from build123d import *

# Parameters (mm, degrees)
SKETCH1_R           = 63.5
SKETCH1_R_2         = 38.1
BOSS_EXTRUDE1_DEPTH = 9.525
SKETCH2_R           = 66.04
SKETCH2_R_2         = 63.5
BOSS_EXTRUDE2_DEPTH = 1.27


with BuildPart() as part:
    # Sketch1 → Boss-Extrude1 (new, symmetric)
    with BuildSketch(Plane.XY):
        with Locations(Location((0, 0, 0), (0, 0, 180))):
            Circle(SKETCH1_R)
        with Locations(Location((0, 0, 0), (0, 0, 180))):
            Circle(SKETCH1_R_2, mode=Mode.SUBTRACT)
    extrude(amount=BOSS_EXTRUDE1_DEPTH, both=True)

    # Sketch2 → Boss-Extrude2 (add, symmetric)
    with BuildSketch(Plane.XY.offset(9.525)):
        Circle(SKETCH2_R)
        with Locations(Location((0, 0, 0), (0, 0, 180))):
            Circle(SKETCH2_R_2, mode=Mode.SUBTRACT)
    extrude(amount=BOSS_EXTRUDE2_DEPTH, both=True)


solid = part.part
Can you work these out from the model? Positions are in its coordinate system, mm. A direction names the side the tool comes from. Give positions to 0.01 mm unless a question says otherwise; leave off trailing zeros. Order: outer loops, then holes, each group sorted by start corner. A loop starts at its lowest first (then second) coordinate and runs counter-clockwise, first axis right, second up. Notation, with made-up numbers: M 42,64.25 L 76,64.25 A17 cw 76,97.25 Z; hole C 34,-17 d3. An arc over 180 degrees is marked long. Use a Markdown table: item, result. Add a question column.
Item 1: For faces 1 (the cylindrical face through (13.77, 61.99, -0.51)), 2 (the flat face through (-27.3, 27.3, -9.525)), 3 (the flat face through (-27.3, 27.3, 9.525)), which set-ups out of +Z, -Z, +X, -X, +Y, -Y let a thin tool reach every point of the face, with its end or its side?
Item 2: If I drill on L1, parallel to Y at x = 0, z = -1.5; L2, parallel to Y at x = 0, z = 9.85; L3, parallel to X at y = 1, z = -1.75, over which ranges is the centre line in solid material (lowest first)? Write a range as [from, to].
Item 3: Will these pins go through, and if not, where does the flat tip stop? pin 1 (5 mm diameter, centred on x = 28, z = -6, fed in from +Y); pin 2 (4 mm diameter, centred on x = -24.5, y = 27.5, fed in from +Z) (3 decimals); pin 3 (4 mm diameter, centred on y = 15, z = -0.5, fed in from +X).
Item 4: Suppose I cut it at A-A (y = 0). List the corners of the cut face in (x, z) for me (3 decimals).
Item 5: Suppose I cut it at C-C (z = 4.5). List the corners of the cut face in (x, y) for me.
Item 6: Suppose I cut it at D-D (y = -56). List the corners of the cut face in (x, z) for me (3 decimals), then the cut area to 3 significant figures.
Item 7: We'd pull the mould along Y, two halves only. Please class faces 4 (the cylindrical face through (8.259, 37.194, -0.133)), 5 (the flat face through (-35, 54, 10.795)), 6 (the cylindrical face through (63, 19.8, 9.5)): +Y half, -Y half, draft (parallel to the pull), parting line (faces both ways), or undercut.
Answer sheet:
| question | item | result |
|---|---|---|
| 1 | face 1 | -Z |
| 1 | face 2 | -Z, +X, -X, +Y, -Y |
| 1 | face 3 | +Z |
| 2 | L1 | y = [-63.5, -38.1], [38.1, 63.5] |
| 2 | L2 | y = [-66.04, -63.5], [63.5, 66.04] |
| 2 | L3 | x = [-63.49, -38.09], [38.09, 63.49] |
| 3 | pin 1 | stops at y = 58.15 |
| 3 | pin 2 | stops at z = 9.525 |
| 3 | pin 3 | stops at x = 62.16 |
| 4 | outline | M -66.04,8.255 L -63.5,8.255 L -63.5,-9.525 L -38.1,-9.525 L -38.1,9.525 L -63.5,9.525 L -63.5,10.795 L -66.04,10.795 Z; M 38.1,-9.525 L 63.5,-9.525 L 63.5,8.255 L 66.04,8.255 L 66.04,10.795 L 63.5,10.795 L 63.5,9.525 L 38.1,9.525 Z |
| 5 | outline | C 0,0 d127; hole C 0,0 d76.2 |
| 6 | outline | M -35.004,8.255 L -29.937,8.255 L -29.937,-9.525 L 29.937,-9.525 L 29.937,8.255 L 35.004,8.255 L 35.004,10.795 L 29.937,10.795 L 29.937,9.525 L -29.937,9.525 L -29.937,10.795 L -35.004,10.795 Z |
| 6 | area | 1,170 mm² |
| 7 | face 4 | undercut |
| 7 | face 5 | draft |
| 7 | face 6 | parting line |
